```python
from build123d import *

# Parameters (mm, degrees)
F_8639_82_80_X_80_X_4_0_1_DEPTH = 2900
SKETCH_3_W                      = 70
SKETCH_3_H                      = 10
CUT_EXTRUDE_1_DEPTH             = 2931.442016311


with BuildPart() as part:
    # Sketch11 → Квадратная труба гост 8639-82 _80 X 80 X 4.0(1) (new body)
    with BuildSketch(Plane(origin=(0, 0, 0), x_dir=(0.4138029443011841, 0.9103664774626047, 0), z_dir=(0.9103664774626047, -0.4138029443011841, 0))):
        with BuildLine():
            Line((-35.999, -40), (35.999, -40))
            ThreePointArc((35.999, -40), (38.828134232, -38.828134232), (40, -35.999))
            Line((40, -35.999), (40, 35.999))
            ThreePointArc((40, 35.999), (38.828134232, 38.828134232), (35.999, 40))
            Line((35.999, 40), (-35.999, 40))
            ThreePointArc((-35.999, 40), (-38.828134232, 38.828134232), (-40, 35.999))
            Line((-40, 35.999), (-40, -35.999))
            ThreePointArc((-40, -35.999), (-38.828134232, -38.828134232), (-35.999, -40))
        make_face()
        with BuildLine():
            Line((-35.999, -36), (35.999, -36))
            ThreePointArc((35.999, -36), (35.999707107, -35.999707107), (36, -35.999))
            Line((36, -35.999), (36, 35.999))
            ThreePointArc((36, 35.999), (35.999707107, 35.999707107), (35.999, 36))
            Line((35.999, 36), (-35.999, 36))
            ThreePointArc((-35.999, 36), (-35.999707107, 35.999707107), (-36, 35.999))
            Line((-36, 35.999), (-36, -35.999))
            ThreePointArc((-36, -35.999), (-35.999707107, -35.999707107), (-35.999, -36))
        make_face(mode=Mode.SUBTRACT)
    extrude(amount=F_8639_82_80_X_80_X_4_0_1_DEPTH)

    # Эскиз3 → Вырез-Вытянуть1 (cut, through all)
    with BuildSketch(Plane(origin=(-16.552117772, -36.414659099, 0), x_dir=(0.9103664774626047, -0.413802944301184, 0), z_dir=(-0.41380294430118403, -0.9103664774626048, 0))):
        with Locations((35, 0)):
            Rectangle(SKETCH_3_W, SKETCH_3_H)
        with Locations((2865, 0)):
            Rectangle(SKETCH_3_W, SKETCH_3_H)
    extrude(amount=-CUT_EXTRUDE_1_DEPTH, mode=Mode.SUBTRACT)


solid = part.part
```
Work out the finished part from the listing and answer in its coordinate system (mm). A direction names the side the tool comes from. Give positions to 0.01 mm unless a question says otherwise; leave off trailing zeros. Write each loop counter-clockwise with the first axis right and the second up, starting at its lowest first coordinate (ties: lowest second). Pieces come first, ordered by that corner, then holes. Notation, with made-up numbers: (22, -30) -> (48, -30) arc R32 cw to (48, 9) -> close; hole circle Ø7 at (7.25, 44.25). An arc over 180 degrees is marked (long way). Write item = value, one per line.
Q1. Section A-A on z = 21 is taken. Determine the outline of the cut face in (x, y), and give its area (3 significant figures).
Computed values:
outline = (-16.55, -36.41) -> (2623.51, -1236.44) -> (2625.17, -1232.8) -> (-14.9, -32.77) -> close; (14.9, 32.77) -> (2654.96, -1167.26) -> (2656.61, -1163.61) -> (16.55, 36.41) -> close
area = 23,200 mm^2
Q2. A tool of negligible diameter and unlimited length cuts with its end or side. For faces 1 (the flat face through (1301, -592, -36)), 2 (the cylindrical face through (1317.63, -556.24, 38.8)), from which of +Z, -Z, +X, -X, +Y, -Y can it reach the whole face along a straight path? Write none if from no direction.
Computed values:
face_1 = none
face_2 = +Z, +X, +Y
Q3. For a pull along X with two mould halves and no side action, classify faces 3 (the flat face through (1302, -591, 40)), 4 (the cylindrical face through (1317.605, -556.295, -38.859)), 5 (the flat face through (1302, -591, 36)) as pulls with the +X half, pulls with the -X half, needs draft (parallel to the pull), parting line crosses it, or undercut.
Computed values:
face_3 = needs draft
face_4 = pulls with the +X half
face_5 = undercut
Q4. Consider line 1 along Z through (x, y) = (277.5, -104); line 2 along Y through (x, z) = (1963, -24.5); line 3 along Y through (x, z) = (1099, 26). Determine where each line is inside the solid, lowest interval first.
Computed values:
line_1 = -40 to -36, 36 to 40
line_2 = -936.21 to -931.82, -852.73 to -848.33
line_3 = -543.48 to -539.09, -460 to -455.61
Q5. Flat-ended cylindrical pins translate along their axes: pin 1 Ø4 at (x, z) = (342, 1.5) entering from +Y; pin 2 Ø1.5 at (x, z) = (319.5, 22) entering from -Y; pin 3 Ø10 at (x, y) = (52, 22) entering from -Z; pin 4 Ø16.5 at (x, y) = (2631.5, -1149) entering from +Z. Find the tip coordinate at first contact, or state that the pin passes through.
Computed values:
pin_1 = -110.61
pin_2 = -189.51
pin_3 = -39.96
pin_4 = 40
